Autodesk Inventor part; units mm, degrees
ref_plane "YZ Plane" through (0, 0, 0) normal (1, 0, 0) x (0, 1, 0)
ref_plane "XZ Plane" through (0, 0, 0) normal (0, 1, 0) x (-1, 0, 0)
ref_plane "XY Plane" through (0, 0, 0) normal (0, 0, 1) x (1, 0, 0)
sketch "Skizze1" plane through (0, 0, 0) normal (0, 0, 1) x (1, 0, 0)
  line L0 (-319.4908, 0) -> (79.1023, 0)
  line L1 (0, -57.6247) -> (0, 149.9482)
  line L2 (17.1489, -27.9715) -> (-12.8511, -27.9715)
  line L3 (-12.8511, -27.9715) -> (-12.8511, 2.0285)
  line L4 (-12.8511, 2.0285) -> (17.1489, 2.0285)
  line L5 (17.1489, 2.0285) -> (17.1489, -27.9715)
  arc A0 (1.933, 106.9528) -> (-27.0148, 99.4639) centre (-12.2357, 102.0285) ccw
  arc A1 (-12.8511, 2.0285) -> (-27.0148, 99.4639) centre (-262.4886, 15.487) ccw
  arc A2 (17.1489, 2.0285) -> (1.933, 106.9528) centre (-262.5489, 15.0327) ccw
  point P0 (0, 0)
  dimension "d0" = 30
  dimension "d1" = 30
  dimension "d2" = 30
  dimension "d4" = 100
  dimension "d6" = 250
  dimension "d7" = 280
extrude "Extrusion1" add sketch "Skizze1" along normal blind 5
sketch "Skizze2" plane through (0, 0, 5) normal (0, 0, 1) x (1, 0, 0)
  arc A0 (1.933, 106.9528) -> (-27.0148, 99.4639) centre (-12.2357, 102.0285) ccw
  point P0 (0, 0)
  dimension "d10" = 0
  dimension "d11" = 0
hole "Bohrung1" at (-12.2357, 102.0285, 5) direction (0, 0, -1) diameter 5 end through all
properties part number "Stütze vorne"
Here's how the part is built. I have some questions about the finished solid (model axes, mm). A direction names the side the tool comes from. Coordinates: 2 decimals unless noted, no trailing zeros. Write each loop counter-clockwise with the first axis right and the second up, starting at its lowest first coordinate (ties: lowest second). Pieces come first, ordered by that corner, then holes.
1) If we section it at C-C (x = -0.5): List the corners of the cut face in (y, z) for me, plus the area to 3 significant figures.
Filled in:
outline: (-27.97, 0) - (111.37, 0) - (111.37, 5) - (-27.97, 5) - close
area: 697 mm2
2) If we section it at B-B (y = -7): List the corners of the cut face in (x, z) for me.
Filled in:
outline: (-12.85, 0) - (17.15, 0) - (17.15, 5) - (-12.85, 5) - close
3) If we section it at A-A (z = 4.2): List the corners of the cut face in (x, y) for me.
Filled in:
outline: (-27.01, 99.46) arc R250 cw to (-12.85, 2.03) - (-12.85, -27.97) - (17.15, -27.97) - (17.15, 2.03) arc R280 ccw to (1.93, 106.95) arc R15 ccw to start; hole circle Ø5 at (-12.24, 102.03)
4) Thinking about a two-plate mould opening in Y: for faces 1 (the face through (-15.19, 52.14, 2.46)), 2 (the face through (-12.346, 104.526, 2.465)), 3 (the face through (0, 46, 0)), 4 (the face through (2, -27.972, 2)), which applies, +Y half, -Y half, draft (parallel to the pull), parting line (faces both ways), or undercut?
Filled in:
face 1: undercut
face 2: undercut
face 3: draft
face 4: -Y half
5) If I drill on line 1 (X direction, y = -19, z = 2.6); line 2 (X direction, y = 25.5, z = 4.2); line 3 (Y direction, x = -8, z = 4.25), over which ranges is the centre line in solid material (lowest first)?
Filled in:
line 1: x = -12.85 to 17.15
line 2: x = -12.69 to 17.26
line 3: y = -27.97 to 116.42
6) Which directions (+Z, -Z, +X, -X, +Y, -Y) give clear straight access to the entire face, cutting with the end or side of a thin tool? Please do faces 5 (the face through (17.149, -13, 2)), 6 (the face through (-12.851, -13, 2)), 7 (the face through (0, 46, 5)).
Filled in:
face 5: +Z, -Z, +X, -Y
face 6: +Z, -Z, -X, -Y
face 7: +Z, +X, -X, +Y, -Y
7) I'm going to push flat-ended pins straight in: pin 1 (1.5 mm diameter, centred on y = -20, z = 3, fed in from +X); pin 2 (2 mm diameter, centred on x = -19.5, z = 1, fed in from +Y). Where does each tip first touch, or does it pass through?
Filled in:
pin 1: stops at x = 17.15
pin 2: stops at y = 115.66
